Check sheet for the drawn part. Datum: minimum x, y, z corner. Units: mm. A direction names the side the tool comes from. Give positions to 0.01 mm unless a question says otherwise; leave off trailing zeros. Order: outer loops, then holes, each group sorted by start corner. A loop starts at its lowest first (then second) coordinate and runs counter-clockwise, first axis right, second up. Notation, with made-up numbers: (29.5, 9) -> (63.5, 9) arc R29 cw to (63.5, 36) -> close; hole circle Ø6 at (85, 36). An arc over 180 degrees is marked (long way). Return JSON: item names as keys, results as strings. Group by question number.
(1) Tool access check on the marked faces 1, 2 and 3. Record the directions out of +Z, -Z, +X, -X, +Y, -Y that give a thin tool (end or side, any length) a straight path to the whole face; none if there is none.
(2) Cross-section at B-B on y = 3.25. Enter the section's corners in (x, z) (1 decimal), then the cut area to 3 significant figures.
(3) Depth check by flat-ended pin: pin 1 Ø2 at (y, z) = (5.5, 20) entering from -X; pin 2 Ø1.5 at (x, y) = (5.5, 8) entering from -Z; pin 3 Ø4 at (y, z) = (4, 14.5) entering from -X. Enter the tip coordinate at first touch or a pass-through.
(4) Cross-section at A-A on x = 20.25. Enter the section's corners in (y, z).
(5) Cross-section at D-D on y = 5.5. Enter the section's corners in (x, z).
(6) Cross-section at C-C on z = 18.75. Enter the section's corners in (x, y).
(7) Thickness scan on line 1 along Z through (x, y) = (12.75, 10); line 2 along Z through (x, y) = (14.75, 7); line 3 along X through (y, z) = (7, 20). Record the ranges inside material, lowest first.
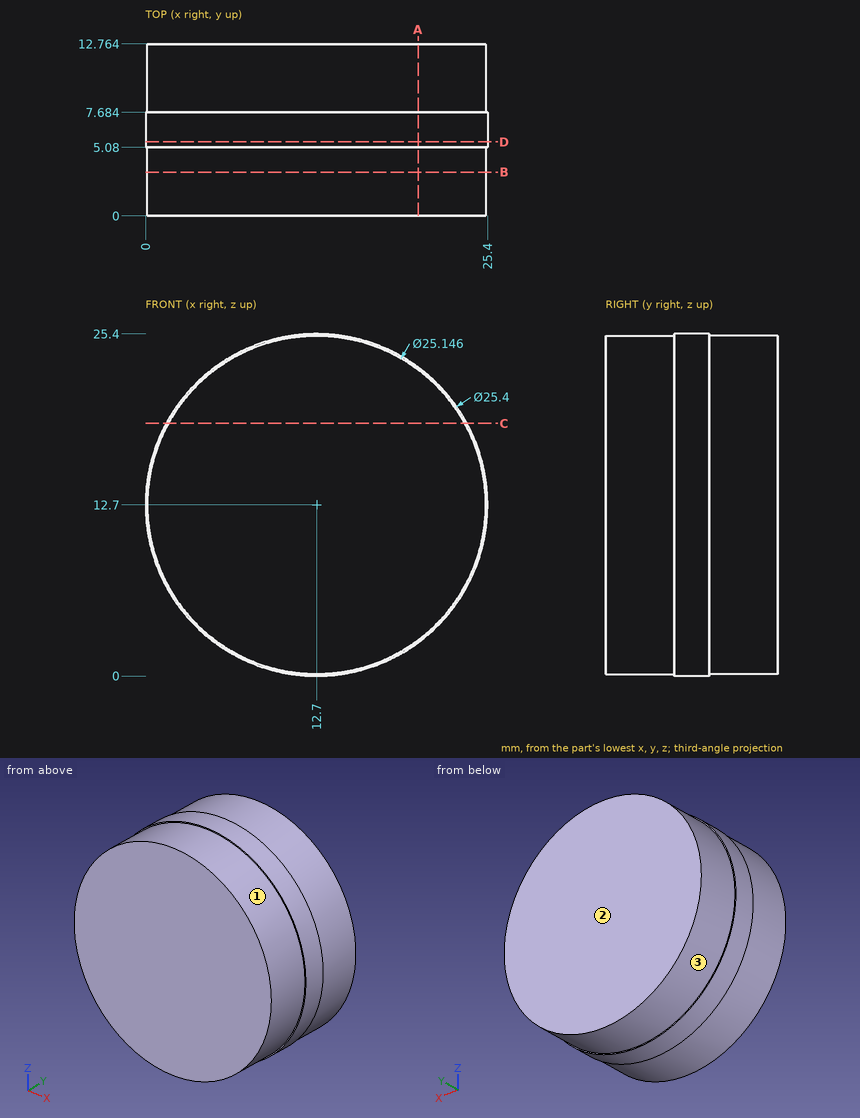
Verdict:
{
 "1": {"face 1": "-Y", "face 2": "+Z, -Z, +X, -X, +Y", "face 3": "+Y"},
 "2": {"outline": "circle Ø25.1 at (12.7, 12.7)", "area": "497 mm²"},
 "3": {"pin 1": "x = 1.67", "pin 2": "z = 1.8", "pin 3": "x = 0"},
 "4": {"outline": "(0, 2.65) -> (5.08, 2.65) -> (5.08, 2.49) -> (7.68, 2.49) -> (7.68, 2.65) -> (12.76, 2.65) -> (12.76, 22.75) -> (7.68, 22.75) -> (7.68, 22.91) -> (5.08, 22.91) -> (5.08, 22.75) -> (0, 22.75) -> close"},
 "5": {"outline": "circle Ø25.4 at (12.7, 12.7)"},
 "6": {"outline": "(1.53, 5.08) -> (1.68, 5.08) -> (1.68, 0) -> (23.72, 0) -> (23.72, 5.08) -> (23.87, 5.08) -> (23.87, 7.68) -> (23.72, 7.68) -> (23.72, 12.76) -> (1.68, 12.76) -> (1.68, 7.68) -> (1.53, 7.68) -> close"},
 "7": {"line 1": "0.13 to 25.27", "line 2": "0.17 to 25.23", "line 3": "2.31 to 23.09"}
}
